from build123d import *

# Parameters (mm, degrees)
SKETCH1_W                = 56
SKETCH1_H                = 13
SKETCH1_W_2              = 13
SKETCH1_H_2              = 45
SKETCH1_H_3              = 5
BOSS_EXTRUDE3_DEPTH      = 49
CUT_EXTRUDE2_DEPTH       = 49
CUT_EXTRUDE3_DEPTH       = 49
SKETCH9_R                = 19
SKETCH9_R_2              = 10
BOSS_EXTRUDE4_DEPTH      = 13
SKETCH11_R               = 19
SKETCH11_R_2             = 10
BOSS_EXTRUDE5_DEPTH      = 13
BOSS_EXTRUDE6_DEPTH      = 58
CUT_EXTRUDE4_DEPTH       = 58
CUT_EXTRUDE5_DEPTH       = 184
BOSS_EXTRUDE7_DEPTH      = 3
BOSS_EXTRUDE7_DEPTH_BACK = 20
SKETCH18_W               = 9.328805748
SKETCH18_H               = 21.574307968
SKETCH18_W_2             = 22.550774564
SKETCH18_H_2             = 22.755980238
CUT_EXTRUDE6_DEPTH       = 535
SKETCH19_R               = 10
CUT_EXTRUDE7_DEPTH       = 29
BOSS_EXTRUDE12_DEPTH     = 284
CUT_EXTRUDE9_DEPTH       = 284
BOSS_EXTRUDE13_DEPTH     = 154
CUT_EXTRUDE12_DEPTH      = 199
CUT_EXTRUDE13_DEPTH      = 73


with BuildPart() as part:
    # Sketch1 → Boss-Extrude3 (new body)
    with BuildSketch(Plane.XY):
        Polygon((0, 82), (0, 75.632885264), (32.75, 56.724663948), (39.25, 67.982994197), (3.742958445, 88.482994197), align=None)
        Polygon((-2.757041555, 77.224663948), (0, 82), (0, 90.643992263), (-0.587168574, 90.982994197), (-7.087168574, 79.724663948), align=None)
        Polygon((0, 90.643992263), (0, 82), (3.742958445, 88.482994197), align=None)
        Polygon((-2.757041555, 77.224663948), (0, 75.632885264), (0, 82), align=None)
        Polygon((39.25, 67.982994197), (32.75, 56.724663948), (44.008330249, 50.224663948), (50.508330249, 61.482994197), align=None)
        Polygon((32.75, 56.724663948), (0, 0), (0, -13), (7.505553499, -13), (44.008330249, 50.224663948), align=None)
        with Locations((-28, -6.5)):
            Rectangle(SKETCH1_W, SKETCH1_H)
        with Locations((-62.5, -6.5)):
            Rectangle(SKETCH1_W_2, SKETCH1_H)
        with Locations((-62.5, 22.5)):
            Rectangle(SKETCH1_W_2, SKETCH1_H_2)
        with Locations((-62.5, 47.5)):
            Rectangle(SKETCH1_W_2, SKETCH1_H_3)
    extrude(amount=BOSS_EXTRUDE3_DEPTH)

    # Sketch5 → Cut-Extrude2 (cut)
    with BuildSketch(Plane.ZY.offset(69)):
        with BuildLine():
            ThreePointArc((24.5, 44), (5.5, 25), (24.5, 6))
            Line((24.5, 6), (24.5, 44))
        make_face()
        with BuildLine():
            Line((24.5, 44), (24.5, 6))
            ThreePointArc((24.5, 6), (37.935028843, 11.564971157), (43.5, 25))
            ThreePointArc((43.5, 25), (37.935028843, 38.435028843), (24.5, 44))
        make_face()
    extrude(amount=-CUT_EXTRUDE2_DEPTH, mode=Mode.SUBTRACT)

    # Sketch6 → Cut-Extrude3 (cut)
    with BuildSketch(Plane(origin=(39.25, 67.982994197, 0), x_dir=(0.866025404, -0.5, 0), z_dir=(0.5, 0.866025404, 0))):
        with BuildLine():
            ThreePointArc((-1.85, -24.5), (-20.85, -5.5), (-39.85, -24.5))
            Line((-39.85, -24.5), (-1.85, -24.5))
        make_face()
        with BuildLine():
            Line((-1.85, -24.5), (-39.85, -24.5))
            ThreePointArc((-39.85, -24.5), (-20.85, -43.5), (-1.85, -24.5))
        make_face()
    extrude(amount=-CUT_EXTRUDE3_DEPTH, mode=Mode.SUBTRACT)

    # Sketch9 → Boss-Extrude4 (add)
    with BuildSketch(Plane(origin=(39.25, 67.982994197, 0), x_dir=(0.866025404, -0.5, 0), z_dir=(0.5, 0.866025404, 0))):
        with Locations((-20.85, -24.5)):
            Circle(SKETCH9_R)
        with Locations((-20.85, -24.5)):
            Circle(SKETCH9_R_2, mode=Mode.SUBTRACT)
    extrude(amount=-BOSS_EXTRUDE4_DEPTH)

    # Sketch11 → Boss-Extrude5 (add)
    with BuildSketch(Plane.ZY.offset(69)):
        with Locations((24.5, 25)):
            Circle(SKETCH11_R)
        with Locations((24.5, 25)):
            Circle(SKETCH11_R_2, mode=Mode.SUBTRACT)
    extrude(amount=-BOSS_EXTRUDE5_DEPTH)

    # Sketch12 → Boss-Extrude6 (add)
    with BuildSketch(Plane.XY.offset(49)):
        with BuildLine():
            Line((50.508330249, 61.482994197), (32.75, 56.724663948))
            ThreePointArc((32.75, 56.724663948), (16.910177277, -16.283097494), (-56, 0))
            Line((-56, 0), (-69, -13))
            ThreePointArc((-69, -13), (22.244773258, -26.285338417), (50.508330249, 61.482994197))
        make_face()
    extrude(amount=-BOSS_EXTRUDE6_DEPTH)

    # Sketch13 → Cut-Extrude4 (cut)
    with BuildSketch(Plane.XY.offset(49)):
        Polygon((32.75, 56.724663948), (39.316517917, 42.098206609), (7.505553499, -13), (-44.392822704, -13), (-56, 0), (0, 0), align=None)
    extrude(amount=-CUT_EXTRUDE4_DEPTH, mode=Mode.SUBTRACT)

    # Sketch16 → Cut-Extrude5 (cut)
    with BuildSketch(Plane.ZY.offset(69)):
        Polygon((-20.067670538, -13), (-20.067670538, 53.233474558), (-20.067670538, 98.990821442), (0, 98.990821442), (0, 53.233474558), (0, -13), (0, -105.844145432), (-20.067670538, -105.844145432), align=None)
    extrude(amount=-CUT_EXTRUDE5_DEPTH, mode=Mode.SUBTRACT)

    # Sketch17 → Boss-Extrude7 (add, two sides)
    with BuildSketch(Plane.ZY.offset(69)) as boss_extrude7_sk:
        with BuildLine():
            ThreePointArc((14.566925199, 26.155), (24.5, 17.31), (34.433074801, 26.155))
            ThreePointArc((34.433074801, 26.155), (24.5, 15), (14.566925199, 26.155))
        make_face()
    extrude(amount=BOSS_EXTRUDE7_DEPTH)
    extrude(boss_extrude7_sk.sketch, amount=-BOSS_EXTRUDE7_DEPTH_BACK)

    # Sketch18 → Cut-Extrude6 (cut)
    with BuildSketch(Plane(origin=(0, 0, 0), x_dir=(-1, 0, 0), z_dir=(0, 0, -1))):
        with Locations((51.335597126, 20.158741433)):
            Rectangle(SKETCH18_W, SKETCH18_H)
        with Locations((80.275387282, 19.567905298)):
            Rectangle(SKETCH18_W_2, SKETCH18_H_2)
    extrude(amount=-CUT_EXTRUDE6_DEPTH, mode=Mode.SUBTRACT)

    # Sketch19 → Cut-Extrude7 (cut)
    with BuildSketch(Plane.ZY.offset(69)):
        with Locations((24.5, 27.31)):
            Circle(SKETCH19_R)
    extrude(amount=-CUT_EXTRUDE7_DEPTH, mode=Mode.SUBTRACT)

    # Sketch21 → Boss-Extrude12 (add)
    with BuildSketch(Plane(origin=(0, 0, 0), x_dir=(-1, 0, 0), z_dir=(0, 0, -1))):
        with BuildLine():
            ThreePointArc((-19.690093366, -27.804633355), (24.032626354, -36.581822551), (64.435496773, -17.705293954))
            Line((64.435496773, -17.705293954), (69, -13))
            Line((69, -13), (56, -13))
            Line((56, -13), (37.73885384, -31.461636701))
            Line((37.73885384, -31.461636701), (34.768910635, -34.431579906))
            Line((34.768910635, -34.431579906), (-19.690093366, -27.804633355))
        make_face()
        with BuildLine():
            Line((37.73885384, -45.225386792), (46.790583005, -35.894459768))
            Line((46.790583005, -35.894459768), (64.435496773, -17.705293954))
            ThreePointArc((64.435496773, -17.705293954), (24.032626354, -36.581822551), (-19.690093366, -27.804633355))
            Line((-19.690093366, -27.804633355), (-22.363127135, -27.479360202))
            Line((-22.363127135, -27.479360202), (-22.615495887, -26.052706761))
            ThreePointArc((-22.615495887, -26.052706761), (-30.437668547, -20.332951122), (-37.413342103, -13.606736129))
            Line((-37.413342103, -13.606736129), (-33.53595077, -35.840606547))
            Line((-33.53595077, -35.840606547), (37.73885384, -45.225386792))
        make_face()
        with BuildLine():
            Line((-48.129988201, 47.84502362), (-37.413342103, -13.606736129))
            ThreePointArc((-37.413342103, -13.606736129), (-30.437668547, -20.332951122), (-22.615495887, -26.052706761))
            Line((-22.615495887, -26.052706761), (-25.567214944, -9.366488243))
            ThreePointArc((-25.567214944, -9.366488243), (-39.428406229, 14.499335876), (-39.316517917, 42.098206609))
            Line((-39.316517917, 42.098206609), (-35.984130282, 49.520865954))
            Line((-35.984130282, 49.520865954), (-36.840667723, 54.362915837))
            Line((-36.840667723, 54.362915837), (-48.129988201, 47.84502362))
        make_face()
        with BuildLine():
            ThreePointArc((-39.316517917, 42.098206609), (-39.428406229, 14.499335876), (-25.567214944, -9.366488243))
            Line((-25.567214944, -9.366488243), (-35.984130282, 49.520865954))
            Line((-35.984130282, 49.520865954), (-39.316517917, 42.098206609))
        make_face()
    extrude(amount=BOSS_EXTRUDE12_DEPTH)

    # Sketch23 → Cut-Extrude9 (cut)
    with BuildSketch(Plane(origin=(0, 0, 0), x_dir=(-1, 0, 0), z_dir=(0, 0, -1))):
        Polygon((56, 0), (-32.75, 56.724663948), (-35.984130282, 49.520865954), (-22.363127135, -27.479360202), (34.768910635, -34.431579906), (56, -13), align=None)
        Polygon((-37.413342103, -13.606736129), (-50.508330249, 61.482994197), (-79.983951007, 56.342705335), (-66.888962861, -18.747024991), align=None)
    extrude(amount=-CUT_EXTRUDE9_DEPTH, mode=Mode.SUBTRACT)

    # Sketch26 → Boss-Extrude13 (add)
    with BuildSketch(Plane.XY):
        with BuildLine():
            ThreePointArc((22.615495887, -26.052706761), (30.437668547, -20.332951122), (37.413342103, -13.606736129))
            Line((37.413342103, -13.606736129), (48.129988201, 47.84502362))
            Line((48.129988201, 47.84502362), (35.984130282, 49.520865954))
            Line((35.984130282, 49.520865954), (22.615495887, -26.052706761))
        make_face()
        with BuildLine():
            Line((-37.73885384, -45.225386792), (33.53595077, -35.840606547))
            Line((33.53595077, -35.840606547), (37.413342103, -13.606736129))
            ThreePointArc((37.413342103, -13.606736129), (30.437668547, -20.332951122), (22.615495887, -26.052706761))
            Line((22.615495887, -26.052706761), (22.363127135, -27.479360202))
            Line((22.363127135, -27.479360202), (19.690093366, -27.804633355))
            ThreePointArc((19.690093366, -27.804633355), (-24.032626354, -36.581822551), (-64.435496773, -17.705293954))
            Line((-64.435496773, -17.705293954), (-37.73885384, -45.225386792))
        make_face()
    extrude(amount=BOSS_EXTRUDE13_DEPTH)

    # Sketch27 → Cut-Extrude12 (cut)
    with BuildSketch(Plane(origin=(39.25, 67.982994197, 0), x_dir=(0.866025404, -0.5, 0), z_dir=(0.5, 0.866025404, 0))):
        Polygon((-46, 0), (13, 0), (177.590878736, 0), (177.590878736, 352.418162382), (13, 352.418162382), (-178.957111939, 352.418162382), (-178.957111939, 168.477547877), (-173.288437482, 168.477547877), (-173.288437482, 0), align=None)
        Polygon((112.21531167, -49), (13, -49), (-46, -49), (-173.288437482, -49), (-173.288437482, -127.513654294), (-173.288437482, -252.662610786), (112.21531167, -252.662610786), (112.21531167, -127.513654294), align=None)
    extrude(amount=-CUT_EXTRUDE12_DEPTH, mode=Mode.SUBTRACT)

    # Sketch28 → Cut-Extrude13 (cut)
    with BuildSketch(Plane.XY.offset(49)):
        Polygon((32.75, 56.724663948), (36.840667723, 54.362915837), (35.984130282, 49.520865954), align=None)
    extrude(amount=-CUT_EXTRUDE13_DEPTH, mode=Mode.SUBTRACT)


solid = part.part
Verification items for the finished model (mm, model axes). A direction names the side the tool comes from. Coordinates: 2 decimals unless noted, no trailing zeros. Write each loop counter-clockwise with the first axis right and the second up, starting at its lowest first coordinate (ties: lowest second). Pieces come first, ordered by that corner, then holes. Notation, with made-up numbers: (62.5, -16.75) -> (108.5, -16.75) arc R13 cw to (108.5, -10.75) -> close; hole circle Ø10 at (1.5, -15.5). An arc over 180 degrees is marked (long way). One line per item, written item: value. Start each with the question number.
Q1. Thickness scan on L1, parallel to Z at x = -61, y = 27; L2, parallel to X at y = 21, z = 41.5; L3, parallel to X at y = 38.5, z = 21.5. Record the ranges inside material, lowest first. Write a range as from..to.
Q2. Mould release check, pull along Y, two halves, no side actions. Record for faces 4 (the flat face through (41.903, 12.14, 24.157)), 5 (the flat face through (31, 12, 49)), 6 (the cylindrical face through (11.606, 76.543, 17.742)): pulls with the +Y half, pulls with the -Y half, needs draft (parallel to the pull), parting line crosses it, or undercut.
Q3. Cross-section at D-D on z = 24.5. Enter the section's corners in (x, y).
Q4. Access from +Z, -Z, +X, -X, +Y, -Y to the whole of each face (thin tool, end or side, straight path). Record for faces 1 (the flat face through (-2.6, -40.6, 24.2)), 2 (the flat face through (-56, 18, 19)), 3 (the flat face through (-63, 50, 24)).
Q5. Go/stop test with flat-tipped pins: P1, Ø8, axis at x = 11, z = 10.5, coming from the +Y side; P2, Ø4, axis at x = -64.5, z = 23, coming from the +Y side; P3, Ø1, axis at y = -31, z = 6.5, coming from the +X side. Record where each tip stops, or that it passes through.
Q6. Cross-section at B-B on z = 45.5. Enter the section's corners in (x, y).
Q7. Cross-section at A-A on y = 23. Enter the section's corners in (x, z).
Q8. Cross-section at C-C on y = 3.5. Enter the section's corners in (x, z).
Checked values:
1. L1: z = 0..14.5, 34.5..49
1. L2: x = -69..-56, 30.94..43.45
1. L3: x = -69..-56, 34.03..46.5
2. face 4: pulls with the -Y half
2. face 5: needs draft
2. face 6: undercut
3. outline: (-69, -13) arc R71.4 ccw to (-64.44, -17.71) -> (-37.74, -45.23) -> (33.54, -35.84) -> (50.51, 61.48) -> (29.85, 73.41) -> (23.35, 62.15) -> (36.84, 54.36) -> (22.36, -27.48) -> (-34.77, -34.43) -> (-56, -13) -> (-56, 17.31) -> (-69, 17.31) -> close; (-69, 37.31) -> (-56, 37.31) -> (-56, 50) -> (-69, 50) -> close; (-7.09, 79.72) -> (6.03, 72.15) -> (12.53, 83.41) -> (-0.59, 90.98) -> close
4. face 1: +Z, -Z, +X, -Y
4. face 2: +Z, -Z, +Y
4. face 3: +Z, -Z, -X, +Y
5. P1: stops at y = 86.6
5. P2: stops at y = 50
5. P3: stops at x = 34.47
6. outline: (-69, -13) arc R71.4 ccw to (-64.44, -17.71) -> (-37.74, -45.23) -> (33.54, -35.84) -> (50.51, 61.48) -> (-0.59, 90.98) -> (-7.09, 79.72) -> (36.84, 54.36) -> (22.36, -27.48) -> (-34.77, -34.43) -> (-56, -13) -> (-56, 50) -> (-69, 50) -> close
7. outline: (-69, 0) -> (-56, 0) -> (-56, 15.48) -> (-69, 15.48) -> close; (-69, 33.52) -> (-56, 33.52) -> (-56, 49) -> (-69, 49) -> close; (31.29, 0) -> (43.8, 0) -> (43.8, 49) -> (31.29, 49) -> close
8. outline: (-69, 0) -> (-56, 0) -> (-56, 49) -> (-69, 49) -> close; (27.84, 0) -> (40.4, 0) -> (40.4, 49) -> (27.84, 49) -> close
